Could you check a few things on this model? Use its own coordinates, in mm. Coordinates: 2 decimals unless noted, no trailing zeros. Order: outer loops, then holes, each group sorted by start corner. A loop starts at its lowest first (then second) coordinate and runs counter-clockwise, first axis right, second up. Notation, with made-up numbers: (-20, 20.25) - (25, 20.25) arc R30 cw to (25, 51.25) - close; hole circle Ø2 at (61, 73.25). An arc over 180 degrees is marked (long way). Answer as a JSON object with one key per item and string values. Group by question number.
(1) Imagine slicing it at A-A, the plane z = -259. Write out the boundary of the cut face in (x, y), and give its area (3 significant figures).
(2) Please list where these lines run through material, in increasing order: probe 1 along Y at (x, z) = (0, -5); probe 2 along X at (y, z) = (0, -13); probe 3 along Z at (x, y) = (0, -6.25).
(3) Imagine slicing it at C-C, the plane x = 9. Write out the boundary of the cut face in (y, z), and give its area (3 significant figures).
(4) Imagine slicing it at B-B, the plane y = -15.5. Write out the boundary of the cut face in (x, z).
(5) Will these pins go through, and if not, where does the flat tip stop? P1, Ø3, axis at y = -2.5, z = -37, coming from the +X side; P2, Ø1.5, axis at y = 4, z = -70.5, coming from the -X side; P3, Ø3, axis at x = 13.5, z = -131, coming from the +Y side.
(6) Imagine slicing it at D-D, the plane x = -14. Write out the boundary of the cut face in (y, z), and give its area (3 significant figures).
from build123d import *

# Parameters (mm, degrees)
SKETCH2_R          = 5
CUT_EXTRUDE1_DEPTH = 328.033828525
SKETCH3_R          = 1.5
CUT_EXTRUDE2_DEPTH = 10


with BuildPart() as part:
    # Sketch1 → Revolve1 (revolve)
    with BuildSketch(Plane(origin=(0, 0, 0), x_dir=(1, 0, 0), z_dir=(0, 1, 0))):
        Polygon((0, 325), (-25.75, 325), (-25.75, 0), (-5, 0), (-5, 25), (0, 25), align=None)
    revolve(axis=Axis((0, 0, -14.83423913), (0, 0, 1)))

    # Sketch2 → Cut-Extrude1 (cut, through all)
    with BuildSketch(Plane(origin=(0, 0, 0), x_dir=(1, 0, 0), z_dir=(0, 1, 0))):
        with Locations(Location((0, 307.5, 0), (0, 0, 270))):
            Circle(SKETCH2_R)
    extrude(amount=-CUT_EXTRUDE1_DEPTH, mode=Mode.SUBTRACT)

    # Sketch3 → Cut-Extrude2 (cut)
    with BuildSketch(Plane.XY):
        with Locations((0, 20)):
            Circle(SKETCH3_R)
    extrude(amount=-CUT_EXTRUDE2_DEPTH, mode=Mode.SUBTRACT)


solid = part.part
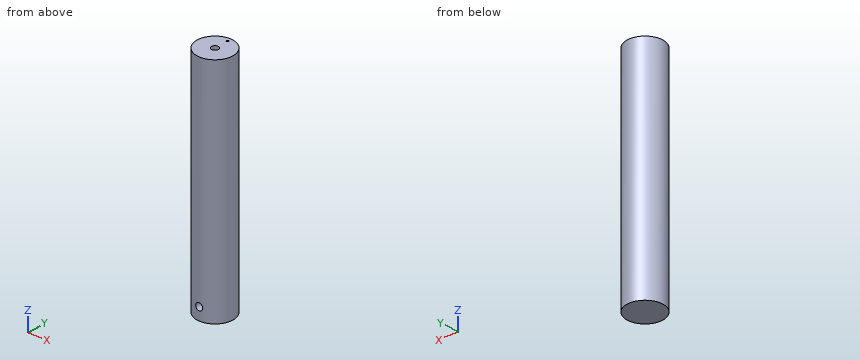
Result set:
{
 "1": {"outline": "circle Ø51.5 at (0, 0)", "area": "2,080 mm^2"},
 "2": {"probe 1": "y = -25.75 to -5, 5 to 18.5, 21.5 to 25.75", "probe 2": "x = -25.75 to -5, 5 to 25.75", "probe 3": "z = -325 to -312.5, -302.5 to 0"},
 "3": {"outline": "(-24.13, -325) - (24.13, -325) - (24.13, 0) - (-24.13, 0) - close", "area": "15,700 mm^2"},
 "4": {"outline": "(-20.56, -325) - (20.56, -325) - (20.56, 0) - (-20.56, 0) - close; hole circle Ø10 at (0, -307.5)"},
 "5": {"P1": "stops at x = 25.73", "P2": "stops at x = -25.54", "P3": "stops at y = 22.78"},
 "6": {"outline": "(-21.61, -325) - (21.61, -325) - (21.61, 0) - (-21.61, 0) - close", "area": "14,000 mm^2"}
}
